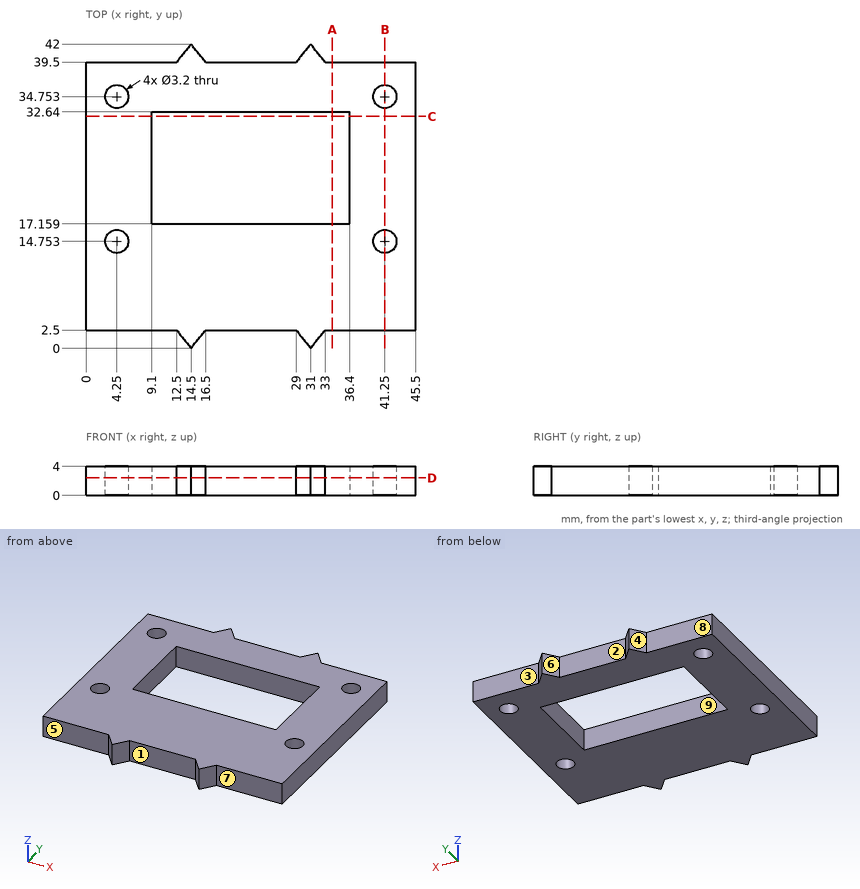
Design review of the part shown in the three views and the two pictorial views. Dimensions are in mm from the part's minimum x, y and z. A direction names the side the tool comes from. Coordinates: 2 decimals unless noted, no trailing zeros. Order: outer loops, then holes, each group sorted by start corner. A loop starts at its lowest first (then second) coordinate and runs counter-clockwise, first axis right, second up. Notation, with made-up numbers: (59.25, 83) -> (116.25, 83) arc R24 ccw to (116.25, 94) -> close; hole circle Ø6 at (46, 44). An arc over 180 degrees is marked (long way). Use one line per item in the form item = value. Start each with the question number.
(1) The part is to be moulded in two halves that separate along X. For the marked faces 1, 2, 3 and 4, say which applies: +X half, -X half, draft (parallel to the pull), parting line (faces both ways), or undercut.
(2) Add section C-C on y = 32. State the section outline as (x, z) points.
(3) For the marked faces 5, 6, 7, 8 and 9, list the 3-axis set-ups (+Z, -Z, +X, -X, +Y, -Y) from which the entire face can be reached by the end or side of a thin tool; tool diameter is ignored.
(4) Add section A-A on x = 34. State the section outline as (y, z) points.
(5) Add section B-B on x = 41.25. State the section outline as (y, z) points.
(6) Insertion check: pin 1 (2.5 mm diameter, centred on x = 41.25, y = 34.75, fed in from +Z); pin 2 (2 mm diameter, centred on x = 37, z = 1.5, fed in from -Y); pin 3 (1 mm diameter, centred on x = 24.5, z = 3.5, fed in from +Y). Each pin has a flat end and moves straight along its axis. Give the tip position at first contact, or say it passes through.
(7) Add section D-D on z = 2.4. State the section outline as (x, y) points, plus the area to 3 significant figures.
(8) For probe 1 along Y at (x, z) = (41.25, 1.8); probe 2 along Y at (x, z) = (18, 2.45); probe 3 along X at (y, z) = (24.5, 3.75), list the stretches that pass through material, from the lowest coordinate up.
Answer block:
q1.face_1 = undercut
q1.face_2 = undercut
q1.face_3 = draft
q1.face_4 = -X half
q2.outline = (0, 0) -> (9.1, 0) -> (9.1, 4) -> (0, 4) -> close; (36.4, 0) -> (45.5, 0) -> (45.5, 4) -> (36.4, 4) -> close
q3.face_5 = +Z, -Z, -X, -Y
q3.face_6 = +Z, -Z, +Y
q3.face_7 = +Z, -Z, +X, -Y
q3.face_8 = +Z, -Z, -X, +Y
q3.face_9 = +Z, -Z
q4.outline = (2.5, 0) -> (17.16, 0) -> (17.16, 4) -> (2.5, 4) -> close; (32.64, 0) -> (39.5, 0) -> (39.5, 4) -> (32.64, 4) -> close
q5.outline = (2.5, 0) -> (13.15, 0) -> (13.15, 4) -> (2.5, 4) -> close; (16.35, 0) -> (33.15, 0) -> (33.15, 4) -> (16.35, 4) -> close; (36.35, 0) -> (39.5, 0) -> (39.5, 4) -> (36.35, 4) -> close
q6.pin_1 = through
q6.pin_2 = 2.5
q6.pin_3 = 39.5
q7.outline = (0, 2.5) -> (12.5, 2.5) -> (14.5, 0) -> (16.5, 2.5) -> (29, 2.5) -> (31, 0) -> (33, 2.5) -> (45.5, 2.5) -> (45.5, 39.5) -> (33, 39.5) -> (31, 42) -> (29, 39.5) -> (16.5, 39.5) -> (14.5, 42) -> (12.5, 39.5) -> (0, 39.5) -> close; hole circle Ø3.2 at (4.25, 14.75); hole circle Ø3.2 at (4.25, 34.75); hole (9.1, 17.16) -> (36.4, 17.16) -> (36.4, 32.64) -> (9.1, 32.64) -> close; hole circle Ø3.2 at (41.25, 14.75); hole circle Ø3.2 at (41.25, 34.75)
q7.area = 1,250 mm²
q8.probe_1 = 2.5 to 13.15, 16.35 to 33.15, 36.35 to 39.5
q8.probe_2 = 2.5 to 17.16, 32.64 to 39.5
q8.probe_3 = 0 to 9.1, 36.4 to 45.5
